Input: dimensioned drawing with shaded views. Units: mm. Origin: part minimum x, y, z. Give positions to 0.01 mm unless a question says otherwise; leave off trailing zeros. Write each loop counter-clockwise with the first axis right and the second up, starting at its lowest first coordinate (ties: lowest second). Pieces come first, ordered by that corner, then holes. Notation, with made-up numbers: M 2.5,74.5 L 38.5,74.5 A13 cw 38.5,93.5 Z; hole C 14.5,62.25 d4. An arc over 180 degrees is marked long. Answer as a JSON object with one key per item and string values.
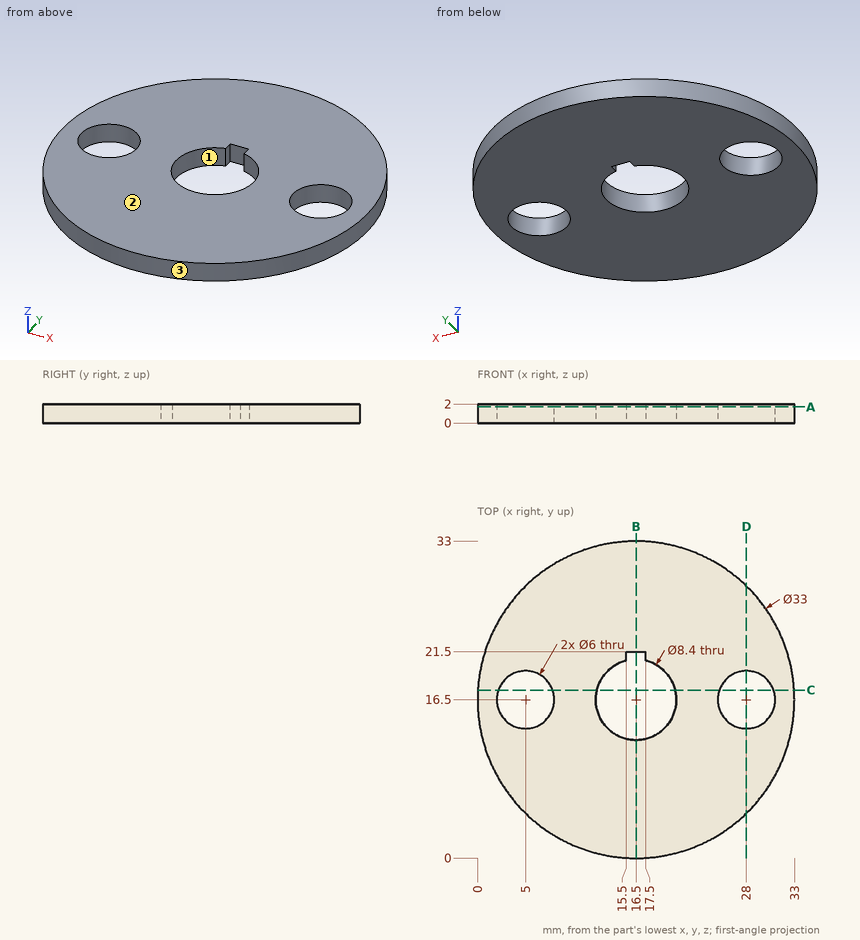
1) Cut plane A-A on z = 1.7. Return loops of the section in (x, y), and give its area (3 significant figures).
Geometry check:
{"outline": "C 16.5,16.5 d33; hole C 5,16.5 d6; hole M 15.5,20.58 A4.2 ccw long 17.5,20.58 L 17.5,21.5 L 15.5,21.5 Z; hole C 28,16.5 d6", "area": "742 mm2"}
2) Cut plane D-D on x = 28. Return loops of the section in (y, z).
Geometry check:
{"outline": "M 4.67,0 L 13.5,0 L 13.5,2 L 4.67,2 Z; M 19.5,0 L 28.33,0 L 28.33,2 L 19.5,2 Z"}
3) Cut plane C-C on y = 17.5. Return loops of the section in (x, z).
Geometry check:
{"outline": "M 0.03,0 L 2.17,0 L 2.17,2 L 0.03,2 Z; M 7.83,0 L 12.42,0 L 12.42,2 L 7.83,2 Z; M 20.58,0 L 25.17,0 L 25.17,2 L 20.58,2 Z; M 30.83,0 L 32.97,0 L 32.97,2 L 30.83,2 Z"}
4) Contact query for flat-ended pins moving along their axis: P1, Ø0.7, axis at y = 21, z = 1, coming from the +X side; P2, Ø1, axis at y = 17.5, z = 0.5, coming from the +X side; P3, Ø1, axis at x = 12, z = 0.5, coming from the +Y side. Output: stop coordinate, or through.
Geometry check:
{"P1": "stops at x = 32.47", "P2": "stops at x = 32.99", "P3": "stops at y = 32.51"}
5) Line query: line 1 (Y direction, x = 16.5, z = 1.5); line 2 (Y direction, x = 7.5, z = 1.1); line 3 (X direction, y = 21, z = 0.25). Output: solid intervals per line, ascending. Write a range as from..to.
Geometry check:
{"line 1": "y = 0..12.3, 21.5..33", "line 2": "y = 2.67..14.84, 18.16..30.33", "line 3": "x = 0.63..15.5, 17.5..32.37"}
6) Pull-direction query (Y, two-part tool) for the marked faces 1, 2 and 3; classes: pulls with the +Y half, pulls with the -Y half, needs draft (parallel to the pull), parting line crosses it, or undercut.
Geometry check:
{"face 1": "undercut", "face 2": "needs draft", "face 3": "parting line crosses it"}
7) Cut plane B-B on x = 16.5. Return loops of the section in (y, z), and give its area (3 significant figures).
Geometry check:
{"outline": "M 0,0 L 12.3,0 L 12.3,2 L 0,2 Z; M 21.5,0 L 33,0 L 33,2 L 21.5,2 Z", "area": "47.6 mm2"}
